Could you check a few things on this drawing? It's one solid part, dimensions in mm from its lowest x, y, z. A direction names the side the tool comes from. Round coordinates to 2 decimals unless told otherwise and drop trailing zeros. Return JSON: item names as keys, results as strings.
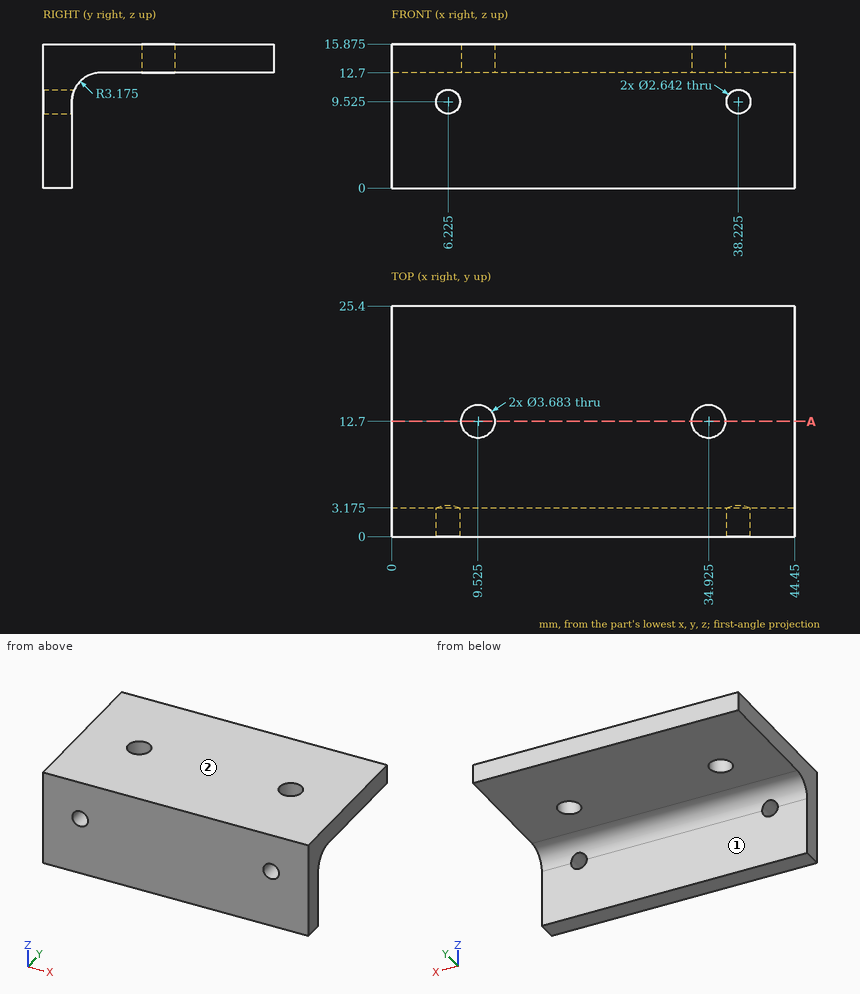
1) I want a section at A-A, the plane y = 12.7. Count the separate pieces of the cut face and the enclosed holes in it, and give its area (3 significant figures).
Return value:
{"separate pieces": "3", "enclosed holes": "0", "area": "118 mm²"}
2) Will these pins go through, and if not, where does the flat tip stop? pin 1 Ø8 at (x, z) = (30.5, 4) entering from +Y (3 decimals); pin 2 Ø5 at (y, z) = (10.5, 10.5) entering from -X; pin 3 Ø9.5 at (x, y) = (23.5, 19.5) entering from -Z.
Return value:
{"pin 1": "y = 3.175", "pin 2": "x = 0", "pin 3": "z = 12.7"}
3) For the marked faces 1 and 2, which set-ups out of +Z, -Z, +X, -X, +Y, -Y let a thin tool reach every point of the face, with its end or its side?
Return value:
{"face 1": "-Z, +X, -X, +Y", "face 2": "+Z, +X, -X, +Y, -Y"}
4) If I drill on probe 1 along X at (y, z) = (12.7, 13.55); probe 2 along Z at (x, y) = (27, 17.75) (1 decimal); probe 3 along Y at (x, z) = (12.5, 9.5) (1 decimal), over which ranges is the centre line in solid material (lowest first)? Write a range as [from, to].
Return value:
{"probe 1": "[0, 7.68], [11.37, 33.08], [36.77, 44.45]", "probe 2": "[12.7, 15.9]", "probe 3": "[0, 3.2]"}
